Source: CAD feature listing. Evaluate the final solid. Frame: model axes, mm. Face numbers are marked on the shaded views. Round coordinates to 2 decimals unless told otherwise and drop trailing zeros. Write each loop counter-clockwise with the first axis right and the second up, starting at its lowest first coordinate (ties: lowest second). Pieces come first, ordered by that corner, then holes. Notation, with made-up numbers: M -14.75,-5 L 44.25,-5 A28 cw 44.25,32 Z; hole C 0,64 d8. An arc over 180 degrees is marked long. Use a Markdown table: item, result.
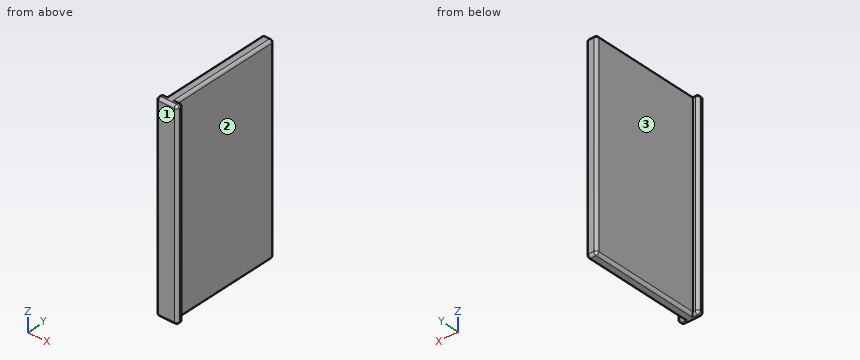
Autodesk Inventor part; units mm, degrees
ref_plane "YZ Plane" through (0, 0, 0) normal (1, 0, 0) x (0, 1, 0)
ref_plane "XZ Plane" through (0, 0, 0) normal (0, 1, 0) x (-1, 0, 0)
ref_plane "XY Plane" through (0, 0, 0) normal (0, 0, 1) x (1, 0, 0)
sketch "Sketch1" plane through (0, 0, 0) normal (0, 0, 1) x (1, 0, 0)
  line L0 (3, 0.8) -> (3, -0.5)
  line L1 (3, -0.5) -> (-1, -0.5)
  line L2 (-1, -0.5) -> (-1, 0.8)
  line L3 (0, 0.8) -> (0, 21.8012)
  line L4 (0, 21.8012) -> (2, 21.8012)
  line L5 (2, 21.8012) -> (2, 0.8)
  line L6 (-1, 0.8) -> (0, 0.8)
  line L7 (2, 0.8) -> (3, 0.8)
  line L8 (-1, 0.8) -> (0, 0.8)
  line L9 (2, 0.8) -> (2.5, 0.8)
  point P0 (0, 0)
  point P1 (1, -0.5)
  point P2 (1, -0.5)
  dimension "d0" = 22.3012
  dimension "d1" = 4
  dimension "d2" = 1.3
  dimension "d3" = 1
  dimension "d4" = 1
extrude "Extrusion1" add sketch "Sketch1" along normal mid plane 37.9984
fillet "Fillet1" radius 0.508 22 edges at (2, 11.3006, 18.9992) (2, 21.8012, 0) (2, 11.3006, -18.9992) (2.5, 0.8, 18.9992) (-0.5, 0.8, 18.9992) (-1, 0.15, 18.9992) (1, -0.5, 18.9992) (3, 0.15, 18.9992) (3, 0.8, 0) (1, 21.8012, 18.9992) (0, 11.3006, 18.9992) (0, 21.8012, 0) (2.5, 0.8, -18.9992) (3, 0.15, -18.9992) (-0.5, 0.8, -18.9992) (-1, 0.15, -18.9992) (1, -0.5, -18.9992) (-1, 0.8, 0) (-1, -0.5, 0) (1, 21.8012, -18.9992) (3, -0.5, 0) (0, 11.3006, -18.9992)
equation "\"d4\" = d3"
properties part number "Medium Conveyor Belt Inserts" material "Acetal Resin, White"
Q1. Mould query, pull axis X, two halves, no side actions, for the marked faces 1, 2 and 3. Classes: +X half, -X half, draft (parallel to the pull), parting line (faces both ways), or undercut.
Results are:
| item | result |
|---|---|
| face 1 | draft |
| face 2 | +X half |
| face 3 | -X half |
Q2. Section A-A on z = -4. Return loops of the section in (x, y), plus the area to 3 significant figures.
Results are:
| item | result |
|---|---|
| outline | M -1,0.01 A0.51 ccw -0.49,-0.5 L 2.49,-0.5 A0.51 ccw 3,0.01 L 3,0.29 A0.51 ccw 2.49,0.8 L 2,0.8 L 2,21.29 A0.51 ccw 1.49,21.8 L 0.51,21.8 A0.51 ccw 0,21.29 L 0,0.8 L -0.49,0.8 A0.51 ccw -1,0.29 Z |
| area | 46.9 mm^2 |
Q3. Line query: L1, parallel to X at y = 5.5, z = 5.5; L2, parallel to Y at x = -0.55, z = 1.5; L3, parallel to Y at x = 0.15, z = -2.5. Output: solid intervals per line, ascending.
Results are:
| item | result |
|---|---|
| L1 | 0 to 2 |
| L2 | -0.5 to 0.8 |
| L3 | -0.5 to 21.65 |
Q4. First-contact query: pin 1 Ø1 at (y, z) = (13, -13.5) entering from -X; pin 2 Ø6 at (y, z) = (10.5, 3) entering from +X; pin 3 Ø0.5 at (x, z) = (0, 8.5) entering from +Y. Flat tips, straight axial feed; report the tip coordinate or a pass-through.
Results are:
| item | result |
|---|---|
| pin 1 | x = 0 |
| pin 2 | x = 2 |
| pin 3 | y = 21.73 |
Q5. Section B-B on y = 18. Return loops of the section in (x, z).
Results are:
| item | result |
|---|---|
| outline | M 0,-18.49 A0.51 ccw 0.51,-19 L 1.49,-19 A0.51 ccw 2,-18.49 L 2,18.49 A0.51 ccw 1.49,19 L 0.51,19 A0.51 ccw 0,18.49 Z |
